The model under review builds one solid part; all positions refer to its coordinate system, in mm. Face numbers are marked on the shaded views. A direction names the side the tool comes from. Give positions to 0.01 mm unless a question says otherwise; leave off trailing zeros. Loops run counter-clockwise (first coordinate to the right, second up) from the corner with the lowest first, then second, coordinate; pieces in that order, holes last. Notation, with made-up numbers: (-19.75, 26) - (-6.75, 26) arc R33 cw to (-6.75, 61) - close; hole circle Ø2 at (-25.75, -22). An arc over 180 degrees is marked (long way). Return JSON: item names as keys, results as strings. Group by question number.
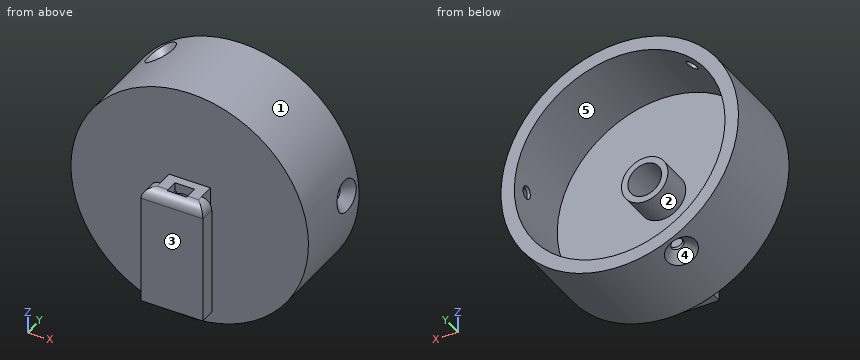
from build123d import *

# Parameters (mm, degrees)
SKETCH1_R           = 23
BOSS_EXTRUDE1_DEPTH = 17
SHELL1_T            = -2.6
SKETCH2_W           = 6
SKETCH2_H           = 23
BOSS_EXTRUDE2_DEPTH = 6
SKETCH3_W           = 2
SKETCH3_H           = 3
CUT_EXTRUDE1_DEPTH  = 50.989999
SKETCH4_R           = 4.5
BOSS_EXTRUDE3_DEPTH = 6
SKETCH5_R           = 3.265
CUT_EXTRUDE2_DEPTH  = 13
SKETCH7_W           = 3.82
SKETCH7_H           = 2.6
CUT_EXTRUDE3_DEPTH  = 1.71
CIRPATTERN1_COUNT   = 3
SKETCH10_W          = 3.1
SKETCH10_H          = 2.2
CUT_EXTRUDE4_DEPTH  = 3
BOSS_EXTRUDE6_REACH = 40.663
SKETCH11_W          = 3.1
SKETCH11_H          = 1.188042875
FILLET1_R           = 2


with BuildPart() as part:
    # Sketch1 → Boss-Extrude1 (new body)
    with BuildSketch(Plane(origin=(0, 0, 0), x_dir=(1, 0, 0), z_dir=(0, 1, 0))):
        with Locations(Location((0, 0, 0), (0, 0, 270))):
            Circle(SKETCH1_R)
    extrude(amount=BOSS_EXTRUDE1_DEPTH)

    # Shell1
    shell1_openings = [part.faces().sort_by_distance(p)[0] for p in [
        (0, 17, 0),
    ]]
    offset(amount=SHELL1_T, openings=shell1_openings, kind=Kind.INTERSECTION)

    # Sketch2 → Boss-Extrude2 (add)
    with BuildSketch(Plane.XZ):
        with Locations((-3, -6.5)):
            Rectangle(SKETCH2_W, SKETCH2_H)
        with Locations((3, -6.5)):
            Rectangle(SKETCH2_W, SKETCH2_H)
    extrude(amount=BOSS_EXTRUDE2_DEPTH)

    # Sketch3 → Cut-Extrude1 (cut, through all)
    with BuildSketch(Plane(origin=(0, 0, -18), x_dir=(-1, 0, 0), z_dir=(0, 0, -1))):
        with Locations((-5, -1.5)):
            Rectangle(SKETCH3_W, SKETCH3_H)
        with Locations((5, -1.5)):
            Rectangle(SKETCH3_W, SKETCH3_H)
    extrude(amount=-CUT_EXTRUDE1_DEPTH, mode=Mode.SUBTRACT)

    # Sketch4 → Boss-Extrude3 (add)
    with BuildSketch(Plane(origin=(0, 2.6, 0), x_dir=(1, 0, 0), z_dir=(0, 1, 0))):
        with Locations(Location((0, 0, 0), (0, 0, 270))):
            Circle(SKETCH4_R)
    extrude(amount=BOSS_EXTRUDE3_DEPTH)

    # Sketch5 → Cut-Extrude2 (cut)
    with BuildSketch(Plane(origin=(0, 8.6, 0), x_dir=(1, 0, 0), z_dir=(0, 1, 0))):
        with Locations(Location((0, 0, 0), (0, 0, 270))):
            Circle(SKETCH5_R)
    extrude(amount=-CUT_EXTRUDE2_DEPTH, mode=Mode.SUBTRACT)

    # Sketch7 → Cut-Extrude3 (cut)
    with BuildSketch(Plane.XY.offset(5)):
        with Locations((0, -3)):
            Rectangle(SKETCH7_W, SKETCH7_H)
    extrude(amount=-CUT_EXTRUDE3_DEPTH, mode=Mode.SUBTRACT)

    # Sketch9 → CSK SLOT for M2 Countersunk Flat Head Screw1 (revolve, cut)
    with BuildSketch(Plane(origin=(22.911051483, 13, 2.020821599), x_dir=(0.08786180866791495, 0, -0.9961326731804369), z_dir=(0, 1, 0))):
        Polygon((0, 0), (0, 5.721032743), (1.2, 5), (1.2, 2), (3.2, 0), align=None)
    csk_slot_for_m2_countersunk_flat_head_sc = revolve(axis=Axis((29.236493958, 13, 2.578744084), (-0.9961326731804366, 0, -0.08786180866791493)), mode=Mode.SUBTRACT)

    # CirPattern1: CSK SLOT for M2 Countersunk Flat Head Screw1 ×3 about axis
    cirpattern1_axis = Axis((0, 17, 0), (0, -1, 0))
    for i in range(1, CIRPATTERN1_COUNT):
        add(csk_slot_for_m2_countersunk_flat_head_sc.rotate(cirpattern1_axis, i * 360 / CIRPATTERN1_COUNT), mode=Mode.SUBTRACT)

    # Sketch10 → Cut-Extrude4 (cut)
    with BuildSketch(Plane.XY.offset(3.29)):
        with Locations((0, -2.8)):
            Rectangle(SKETCH10_W, SKETCH10_H)
    extrude(amount=-CUT_EXTRUDE4_DEPTH, mode=Mode.SUBTRACT)

    # Sketch11 → Boss-Extrude6 (add, up to next)
    with BuildSketch(Plane(origin=(0, -3.9, 0), x_dir=(1, 0, 0), z_dir=(0, 1, 0)), mode=Mode.PRIVATE) as boss_extrude6_sk1:
        with Locations((0, -2.695978563)):
            Rectangle(SKETCH11_W, SKETCH11_H)
    boss_extrude6_tool1 = extrude(boss_extrude6_sk1.sketch, amount=-BOSS_EXTRUDE6_REACH, mode=Mode.PRIVATE) - part.part
    add(boss_extrude6_tool1.solids().sort_by_distance((0, -3.9, 2.695979))[0])

    # Fillet1
    # the kernel refuses this fillet: 2 mm, written as the material it takes off along each edge
    with BuildSketch(Plane(origin=(-6, 2, 5), x_dir=(1, 0, 0), z_dir=(0, -1, 0))) as fillet1_piece_1_section:
        with BuildLine():
            CenterArc((FILLET1_R, -FILLET1_R), FILLET1_R, 90, 90)
            Line((0, -FILLET1_R), (0, 0))
            Line((0, 0), (FILLET1_R, 0))
        make_face()
    fillet1_piece_1 = extrude(amount=13, mode=Mode.PRIVATE)
    fillet1_piece_1 = split(fillet1_piece_1, bisect_by=Plane(origin=(-5.547209771, 0, 4.547209771), z_dir=(0, -1, 0)), keep=Keep.TOP, mode=Mode.PRIVATE)
    add(fillet1_piece_1, mode=Mode.SUBTRACT)
    with BuildSketch(Plane(origin=(-11, -6, 5), x_dir=(0, 1, 0), z_dir=(1, 0, 0))) as fillet1_piece_2:
        with BuildLine():
            CenterArc((FILLET1_R, -FILLET1_R), FILLET1_R, 90, 90)
            Line((0, -FILLET1_R), (0, 0))
            Line((0, 0), (FILLET1_R, 0))
        make_face()
    extrude(amount=22, mode=Mode.SUBTRACT)
    with BuildSketch(Plane(origin=(6, 2, 5), x_dir=(-1, 0, 0), z_dir=(0, -1, 0))) as fillet1_piece_3_section:
        with BuildLine():
            CenterArc((FILLET1_R, FILLET1_R), FILLET1_R, 180, 90)
            Line((0, FILLET1_R), (0, 0))
            Line((0, 0), (FILLET1_R, 0))
        make_face()
    fillet1_piece_3 = extrude(amount=13, mode=Mode.PRIVATE)
    fillet1_piece_3 = split(fillet1_piece_3, bisect_by=Plane(origin=(5.547209771, 0, 4.547209771), z_dir=(0, -1, 0)), keep=Keep.TOP, mode=Mode.PRIVATE)
    add(fillet1_piece_3, mode=Mode.SUBTRACT)


solid = part.part
Item 1: Mouldability with a two-part tool opening along X and no side actions: class the marked faces 1, 2 and 3 as +X half, -X half, draft (parallel to the pull), parting line (faces both ways), or undercut.
Item 2: For P1, Ø2.5, axis at y = -1.5, z = -8, coming from the +X side; P2, Ø1.9, axis at y = -3.5, z = 4, coming from the +X side; P3, Ø6, axis at y = 2, z = -10.5, coming from the +X side; P4, Ø4.5, axis at x = 0.5, y = -2, coming from the +Z side, all flat-tipped, find the tip position at first contact; note any pin that passes through.
Item 3: Tool access review of the marked faces 4 and 5: name each direction out of +Z, -Z, +X, -X, +Y, -Y from which nothing blocks a thin tool from reaching the whole face with its end or side.
Item 4: For L1, parallel to X at y = 5.25, z = 0 (3 decimals); L2, parallel to X at y = 9.25, z = 0; L3, parallel to Y at x = -7, z = 16, list the stretches that pass through material, from the lowest coordinate up. Write a range as from..to.
Item 5: Take a section at C-C (y = 3.5). State the section outline as (x, z) points (3 decimals), then the cut area to 3 significant figures.
Item 6: Take a section at B-B (y = -1). State the section outline as (x, z) points (3 decimals).
Item 7: Take a section at A-A (x = 0). State the section outline as (y, z) points (3 decimals).
Item 8: Take a section at D-D (z = -14). State the section outline as (x, y) points.
Check sheet entries:
{
 "1": {"face 1": "parting line", "face 2": "undercut", "face 3": "draft"},
 "2": {"P1": "stops at x = 4", "P2": "stops at x = 6", "P3": "stops at x = 21.74", "P4": "stops at z = 23"},
 "3": {"face 4": "-Z", "face 5": "+Y"},
 "4": {"L1": "x = -23..-20.4, -4.5..-3.265, 3.265..4.5, 20.4..23", "L2": "x = -23..-20.4, 20.4..23", "L3": "y = 0..2.6"},
 "5": {"outline": "circle Ø46 at (0, 0); circle Ø9 at (0, 0); hole circle Ø40.8 at (0, 0); hole circle Ø6.53 at (0, 0)", "area": "385 mm^2"},
 "6": {"outline": "(-4, -18) - (4, -18) - (4, 5) - (-4, 5) - close; hole circle Ø6.53 at (0, 0)"},
 "7": {"outline": "(-6, -18) - (0, -18) - (0, -23) - (17, -23) - (17, -20.4) - (2.6, -20.4) - (2.6, -4.5) - (8.6, -4.5) - (8.6, -3.265) - (-4.4, -3.265) - (-4.4, 2.102) - (-3.9, 2.102) - (-3.9, 3.29) - (-4.3, 3.29) - (-4.3, 4.977) arc R2 ccw to (-6, 3) - close; (-1.7, 3.265) - (8.6, 3.265) - (8.6, 4.5) - (2.6, 4.5) - (2.6, 20.4) - (17, 20.4) - (17, 23) - (0, 23) - (0, 5) - (-1.7, 5) - close"},
 "8": {"outline": "(-18.25, 0) - (-4, 0) - (-4, -3) - (-6, -3) - (-6, -6) - (6, -6) - (6, -3) - (4, -3) - (4, 0) - (18.25, 0) - (18.25, 17) - (14.84, 17) - (14.84, 2.6) - (-14.84, 2.6) - (-14.84, 17) - (-18.25, 17) - close"}
}
